Read the model definition and answer for the solid it produces. Units are mm, in the model's axes. A direction names the side the tool comes from. Give positions to 0.01 mm unless a question says otherwise; leave off trailing zeros. Write each loop counter-clockwise with the first axis right and the second up, starting at its lowest first coordinate (ties: lowest second). Pieces come first, ordered by that corner, then holes. Notation, with made-up numbers: (-5, 54) -> (18, 54) arc R16 ccw to (18, 67) -> close; hole circle Ø10 at (79.25, -19). An arc over 180 degrees is marked (long way). Use a Markdown table: item, result.
from build123d import *

# Parameters (mm, degrees)
BASE_FLANGE1_DEPTH       = 0.7366
SKETCHED_START           = -24.545942999
SKETCHED_BEND1_OUTLINE_W = 0.7366
SKETCHED_BEND1_OUTLINE_H = 40
SKETCHED_BEND1_DEPTH     = 45.545942999
SKETCHED_START_2         = -25.131186431
SKETCHED_BEND1_2_DEPTH   = 0.004036568
SKETCHED_START_3         = -25.867786431
SKETCHED_BEND1_3_DEPTH   = 1.4732
SKETCHED_START_4         = -20
SKETCHED_BEND1_4_DEPTH   = 40
M3_CLEARANCE_HOLE1_D     = 3.4
M3_CLEARANCE_HOLE1_DEPTH = 0.7366
M3_CLEARANCE_HOLE1_TIP   = 1.021463052


with BuildPart() as part:
    # Base-Flange1: sheet metal written as solids
    # Sketch1 → Base-Flange1 (new body)
    with BuildSketch(Plane.YZ):
        with BuildLine():
            Line((-20, 0), (-20, -95))
            ThreePointArc((-20, -95), (-18.535533906, -98.535533906), (-15, -100))
            Line((-15, -100), (15, -100))
            ThreePointArc((15, -100), (18.535533906, -98.535533906), (20, -95))
            Line((20, -95), (20, 0))
            ThreePointArc((20, 0), (0, 20), (-20, 0))
        make_face()
    extrude(amount=-BASE_FLANGE1_DEPTH)

    # Sketched Bend1: read off the stored shape, not the designer's step
    # Sketched Bend1 outline → Sketched Bend1 (cut)
    with BuildSketch(Plane.XY.offset(SKETCHED_START)):
        with Locations((-0.3683, 0)):
            Rectangle(SKETCHED_BEND1_OUTLINE_W, SKETCHED_BEND1_OUTLINE_H)
    extrude(amount=SKETCHED_BEND1_DEPTH, mode=Mode.SUBTRACT)

    # Sketched Bend1 2 outline → Sketched Bend1 2 (add)
    with BuildSketch(Plane.XY.offset(SKETCHED_START_2)):
        with BuildLine():
            ThreePointArc((24.868813569, -20), (44.868813569, 0), (24.868813569, 20))
            Line((24.868813569, 20), (0, 20))
            Line((0, 20), (0, -20))
            Line((0, -20), (24.868813569, -20))
        make_face()
    extrude(amount=SKETCHED_BEND1_2_DEPTH)

    # Sketched Bend1 3 outline → Sketched Bend1 3 (add)
    with BuildSketch(Plane.XY.offset(SKETCHED_START_3)):
        with BuildLine():
            ThreePointArc((24.868813569, -20), (44.868813569, 0), (24.868813569, 20))
            Line((24.868813569, 20), (0, 20))
            Line((0, 20), (0, -20))
            Line((0, -20), (24.868813569, -20))
        make_face()
    extrude(amount=SKETCHED_BEND1_3_DEPTH)

    # Sketched Bend1 4 outline → Sketched Bend1 4 (cut)
    with BuildSketch(Plane(origin=(0, 0, 0), x_dir=(1, 0, 0), z_dir=(0, 1, 0)).offset(SKETCHED_START_4)):
        with BuildLine():
            ThreePointArc((0, 25.867786431), (0.215745145, 25.346931576), (0.7366, 25.131186431))
            Line((0.7366, 25.131186431), (46, 25.131186431))
            Line((46, 25.131186431), (46, 25.867786431))
            Line((46, 25.867786431), (0, 25.867786431))
        make_face()
        with BuildLine():
            Line((46, 23), (46, 24.394586426))
            Line((46, 24.394586426), (0.7366, 24.394586431))
            ThreePointArc((0.7366, 24.394586431), (-0.30510971, 24.826076721), (-0.7366, 25.867786431))
            Line((-0.7366, 25.867786431), (-0.7366, 27))
            Line((-0.7366, 27), (-2, 27))
            Line((-2, 27), (-2, 24.545942999))
            Line((-2, 24.545942999), (0, 24.545942999))
            Line((0, 24.545942999), (0, 23))
            Line((0, 23), (46, 23))
        make_face()
    extrude(amount=SKETCHED_BEND1_4_DEPTH, mode=Mode.SUBTRACT)

    # M3 Clearance Hole1
    with Locations(Plane(origin=(0, 0, -24.394586431), x_dir=(0, -1, 0), z_dir=(0, 0, 1))):
        with Locations((0, 37.368813569), (-12.5, 24.868813569), (0, 12.368813569), (12.5, 24.868813569)):
            Hole(M3_CLEARANCE_HOLE1_D / 2, depth=M3_CLEARANCE_HOLE1_DEPTH)
            with Locations((0, 0, -(M3_CLEARANCE_HOLE1_DEPTH + M3_CLEARANCE_HOLE1_TIP / 2))):  # 118° drill point
                Cone(0, M3_CLEARANCE_HOLE1_D / 2, M3_CLEARANCE_HOLE1_TIP, mode=Mode.SUBTRACT)


solid = part.part
Item 1: For a pull along Y with two mould halves and no side action, classify faces 3 (the face through (-0.29, -0.28, -24.81)), 4 (the face through (44.864, -0.44, -24.768)), 5 (the face through (23.36, 13.28, -24.77)) as +Y half, -Y half, draft (parallel to the pull), parting line (faces both ways), or undercut.
Return value:
| item | result |
|---|---|
| face 3 | draft |
| face 4 | parting line |
| face 5 | undercut |
Item 2: Each of these flat-tipped pins is pushed along its axis until it touches: P1, Ø2, axis at x = 37.37, y = 0, coming from the -Z side; P2, Ø4, axis at x = 27.5, y = -6.5, coming from the -Z side; P3, Ø20, axis at y = -8.5, z = -79, coming from the +X side. Where does it stop, or does it pass through?
Return value:
| item | result |
|---|---|
| P1 | through |
| P2 | z = -25.13 |
| P3 | x = 0 |
Item 3: A cutting plane is placed at D-D (x = 3). Give the vertices of the cut face in (y, z), then the cut area to 3 significant figures.
Return value:
| item | result |
|---|---|
| outline | (-20, -25.13) -> (20, -25.13) -> (20, -24.39) -> (-20, -24.39) -> close |
| area | 29.5 mm^2 |
Item 4: A cutting plane is placed at B-B (y = -12.5). Give the vertices of the cut face in (x, z).
Return value:
| item | result |
|---|---|
| outline | (-0.74, -100) -> (0, -100) -> (0, -25.87) arc R0.74 cw to (0.74, -25.13) -> (23.17, -25.13) -> (23.17, -24.39) -> (0.74, -24.39) arc R1.47 ccw to (-0.74, -25.87) -> close; (26.57, -25.13) -> (40.48, -25.13) -> (40.48, -24.39) -> (26.57, -24.39) -> close |
Item 5: Straight lines are drawn through the part: line 1 along X through (y, z) = (0, -24.8); line 2 along Z through (x, y) = (41.5, 3.5); line 3 along X through (y, z) = (5.5, -75.5). For each, find the intervals that lie inside material, in ascending order. Write a range as [from, to].
Return value:
| item | result |
|---|---|
| line 1 | [-0.28, 10.67], [14.07, 35.67], [39.07, 44.87] |
| line 2 | [-25.13, -24.39] |
| line 3 | [-0.74, 0] |
Item 6: A cutting plane is placed at A-A (y = 0). Give the vertices of the cut face in (x, z).
Return value:
| item | result |
|---|---|
| outline | (-0.74, -100) -> (0, -100) -> (0, -25.87) arc R0.74 cw to (0.74, -25.13) -> (10.67, -25.13) -> (10.67, -24.39) -> (0.74, -24.39) arc R1.47 ccw to (-0.74, -25.87) -> close; (14.07, -25.13) -> (35.67, -25.13) -> (35.67, -24.39) -> (14.07, -24.39) -> close; (39.07, -25.13) -> (44.87, -25.13) -> (44.87, -24.39) -> (39.07, -24.39) -> close |
Item 7: A cutting plane is placed at C-C (z = -82.5). Give the vertices of the cut face in (x, y).
Return value:
| item | result |
|---|---|
| outline | (-0.74, -20) -> (0, -20) -> (0, 20) -> (-0.74, 20) -> close |
Item 8: A tool of negligible diameter and unlimited length cuts with its end or side. For faces 1 (the face through (0, 0, -62)), 2 (the face through (-0.36, 18.5, -98.57)), from which of +Z, -Z, +X, -X, +Y, -Y can it reach the whole face along a straight path? Write none if from no direction.
Return value:
| item | result |
|---|---|
| face 1 | -Z, +X, +Y, -Y |
| face 2 | -Z, +X, -X, +Y |
